Could you check a few things on this model? Use its own coordinates, in mm. Round coordinates to 2 decimals unless told otherwise and drop trailing zeros. Write each loop counter-clockwise with the first axis right and the second up, starting at its lowest first coordinate (ties: lowest second). Pieces come first, ordered by that corner, then holes. Notation, with made-up numbers: (-10.75, 51.25) -> (1.25, 51.25) arc R7 cw to (1.25, 56.25) -> close; hole circle Ø10 at (-14.5, -11.5). An arc over 180 degrees is marked (long way). Answer in a Markdown table with one row per item.
Autodesk Inventor part; units mm, degrees
ref_plane "YZ Plane" through (0, 0, 0) normal (1, 0, 0) x (0, 1, 0)
ref_plane "XZ Plane" through (0, 0, 0) normal (0, 1, 0) x (-1, 0, 0)
ref_plane "XY Plane" through (0, 0, 0) normal (0, 0, 1) x (1, 0, 0)
sketch "スケッチ1" plane through (0, 0, 0) normal (0, 1, 0) x (-1, 0, 0)
  line L0 (148.5, 200.09) -> (-148.5, 200.09)
  line L1 (-148.5, 200.09) -> (-148.5, -200.09)
  line L2 (-148.5, -200.09) -> (148.5, -200.09)
  line L3 (148.5, -200.09) -> (148.5, 200.09)
  line L4 (148.5, 200.09) -> (-148.5, -200.09) construction
  line L5 (-148.5, 200.09) -> (148.5, -200.09) construction
  line L6 (-148.5, 190.77) -> (148.5, 190.77)
  line L7 (-207.9, 0) -> (207.9, 0) construction
  line L8 (-148.5, -190.77) -> (148.5, -190.77)
  line L9 (-148.5, 200) -> (148.5, 200)
  line L10 (-148.5, -200) -> (148.5, -200)
  point P0 (0, 0)
  point P1 (-148.5, -200)
  point P2 (-148.5, -190.77)
  dimension "d1" = 297
  dimension "d4" = 9.32
  dimension "d5" = 0.09
  dimension "d10" = 400
extrude "押し出し1" add sketch "スケッチ1" along normal blind 0.09
extrude "押し出し2" add sketch "スケッチ1" against normal blind 0.5 contours L3 L9 L1 L0 | L3 L2 L1 L10
extrude "押し出し3" add sketch "スケッチ1" against normal blind 0.09 from surface at -0.5 contours L3 L9 L1 L0 | L3 L6 L1 L9 | L3 L10 L1 L8 | L3 L2 L1 L10
properties part number "field_plate_SUS4301"
1) Imagine slicing it at C-C, the plane z = -49. Please give me the cut outline in (x, y), plus the area to 3 significant figures.
Findings:
| item | result |
|---|---|
| outline | (-148.5, 0) -> (148.5, 0) -> (148.5, 0.09) -> (-148.5, 0.09) -> close |
| area | 26.7 mm^2 |
2) Imagine slicing it at B-B, the plane x = 24.5. Please give me the cut outline in (y, z).
Findings:
| item | result |
|---|---|
| outline | (-0.59, -200.09) -> (0.09, -200.09) -> (0.09, 200.09) -> (-0.59, 200.09) -> (-0.59, 190.77) -> (-0.5, 190.77) -> (-0.5, 200) -> (0, 200) -> (0, -200) -> (-0.5, -200) -> (-0.5, -190.77) -> (-0.59, -190.77) -> close |
3) Imagine slicing it at A-A, the plane y = -0.35. Please give me the cut outline in (x, z), plus the area to 3 significant figures.
Findings:
| item | result |
|---|---|
| outline | (-148.5, -200.09) -> (148.5, -200.09) -> (148.5, -200) -> (-148.5, -200) -> close; (-148.5, 200) -> (148.5, 200) -> (148.5, 200.09) -> (-148.5, 200.09) -> close |
| area | 53.5 mm^2 |
4) For pin 1 (2 mm diameter, centred on x = -12, z = -13.5, fed in from -Y), with a flat end and sliding along its axis, tell me the tip position at first contact or that it passes through.
Findings:
| item | result |
|---|---|
| pin 1 | stops at y = 0 |
